Input: dimensioned drawing with shaded views. Units: mm. Origin: part minimum x, y, z. Coordinates: 2 decimals unless noted, no trailing zeros. Write each loop counter-clockwise with the first axis right and the second up, starting at its lowest first coordinate (ties: lowest second). Pieces come first, ordered by that corner, then holes. Notation, with made-up numbers: (70.5, -37) -> (90.5, -37) arc R26 cw to (90.5, -2) -> close; hole circle Ø5 at (-14.75, 48.5). An arc over 180 degrees is marked (long way). One line per item, written item: value. Start each with the question number.
1. First-contact query: P1, Ø1.8, axis at y = 2, z = 5.85, coming from the +X side. Flat tip, straight axial feed; report the tip coordinate or a pass-through.
2. Section query A-A, the plane y = 11.25. Output: boundary loops of the cut face in (x, z) (1 decimal).
3. Section query B-B, the plane z = 17.75. Output: boundary loops of the cut face in (x, y) (1 decimal).
4. Section query C-C, the plane y = 2. State how many separate pieces and enclosed holes the cut face has.
5. Line query: line 1 (Z direction, x = 0.7, y = 2.5) (1 decimal); line 2 (Y direction, x = 0.3, z = 13.25) (1 decimal); line 3 (Y direction, x = 0.1, z = 13.75) (1 decimal). Output: solid intervals per line, ascending.
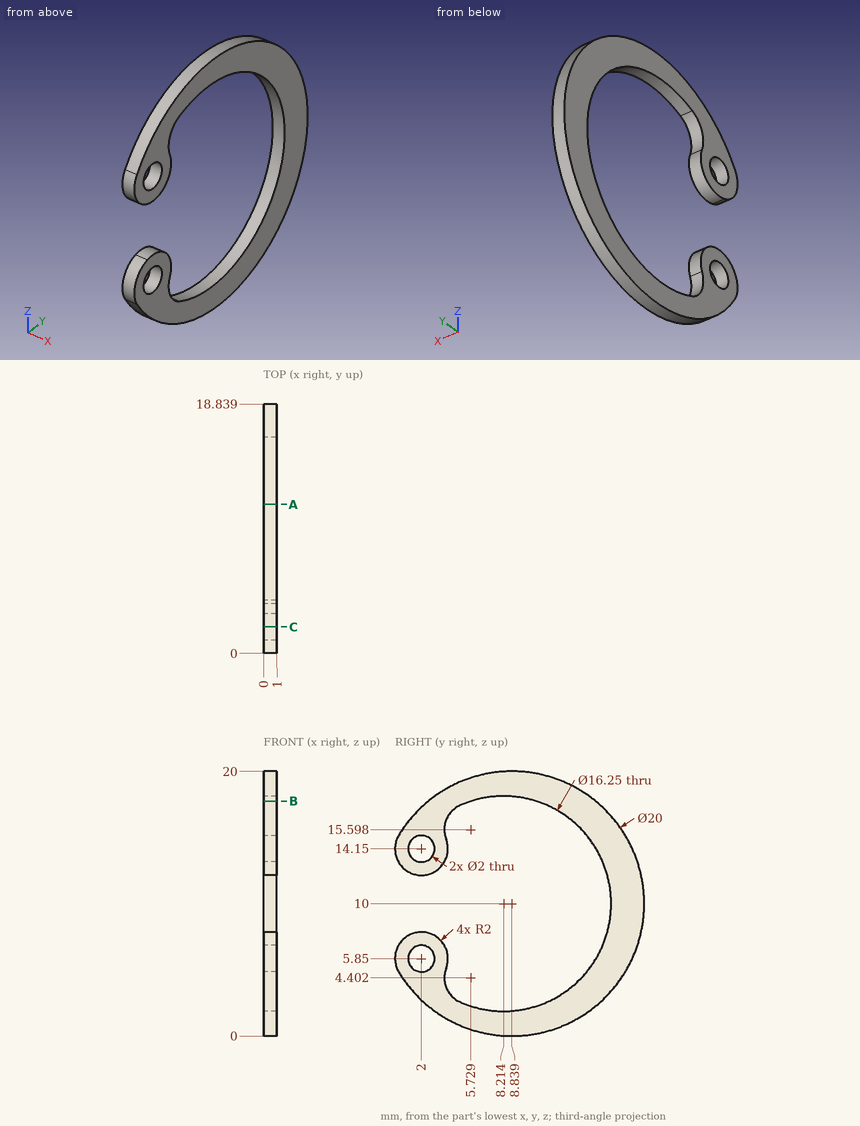
Computed values:
1. P1: passes through
2. outline: (0, 0.3) -> (1, 0.3) -> (1, 2.5) -> (0, 2.5) -> close; (0, 17.5) -> (1, 17.5) -> (1, 19.7) -> (0, 19.7) -> close
3. outline: (0, 2.5) -> (1, 2.5) -> (1, 5.8) -> (0, 5.8) -> close; (0, 10.7) -> (1, 10.7) -> (1, 15.2) -> (0, 15.2) -> close
4. separate pieces: 4
4. enclosed holes: 0
5. line 1: z = 2.3 to 5, 6.7 to 7.8, 12.2 to 13.3, 15 to 17.7
5. line 2: y = 0.2 to 1.6, 2.4 to 3.8, 15.7 to 18.3
5. line 3: y = 0 to 1.1, 2.9 to 4, 15.4 to 18.1
